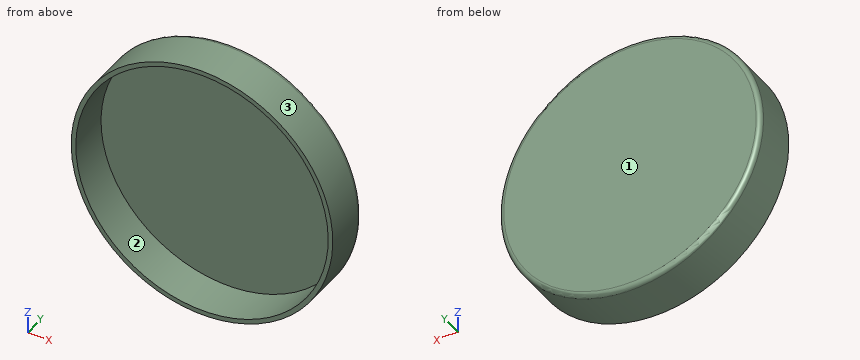
```python
from build123d import *

# Parameters (mm, degrees)
ESQUISSE1_R        = 14.3
BOSS_EXTRU_1_DEPTH = 5
COQUE1_T           = -0.5
CONG_1_R           = 0.5


with BuildPart() as part:
    # Esquisse1 → Boss.-Extru.1 (new body)
    with BuildSketch(Plane(origin=(0, 0, 0), x_dir=(1, 0, 0), z_dir=(0, 1, 0))):
        with Locations(Location((0, 0, 0), (0, 0, 270))):
            Circle(ESQUISSE1_R)
    extrude(amount=BOSS_EXTRU_1_DEPTH)

    # Coque1
    coque1_openings = [part.faces().sort_by_distance(p)[0] for p in [
        (0, 0, 0),
    ]]
    offset(amount=COQUE1_T, openings=coque1_openings, kind=Kind.INTERSECTION)

    # Congé1
    cong_1_edges = [part.edges().sort_by_distance(p)[0] for p in [
        (0, 5, -14.3),
    ]]
    fillet(cong_1_edges, radius=CONG_1_R)


solid = part.part
```
Can you work these out from the model? Positions are in its coordinate system, mm. Face numbers are marked on the shaded views. Give positions to 0.01 mm unless a question says otherwise; leave off trailing zeros. Loops run counter-clockwise (first coordinate to the right, second up) from the corner with the lowest first, then second, coordinate; pieces in that order, holes last. Notation, with made-up numbers: M 78.5,50 L 111.5,50 A24 ccw 111.5,74 Z; hole C 1.25,84 d10. An arc over 180 degrees is marked long. Use CSV: the item, a comma, the result in double quotes. Start each with the question number.
1. Imagine slicing it at C-C, the plane x = 0. Write out the boundary of the cut face in (y, z), plus the area to 3 significant figures.
2. If I drill on L1, parallel to X at y = 1.65, z = 0; L2, parallel to Y at x = -9, z = -5; L3, parallel to X at y = 1.35, z = 9, over which ranges is the centre line in solid material (lowest first)?
3. Imagine slicing it at A-A, the plane z = 0. Write out the boundary of the cut face in (x, y), plus the area to 3 significant figures.
4. If we mould it in two halves opening along X, with no side actions, what happens to the marked faces 1, 2 and 3? For each: released by +X, released by -X, zero draft, split by the parting line, or undercut.
5. For P1, Ø2, axis at x = -9, y = 2.5, coming from the +Z side; P2, Ø1.5, axis at x = 4, y = 3, coming from the -Z side; P3, Ø3, axis at y = 3, z = -3.5, coming from the +X side, each with a flat end and sliding along its axis, tell me the tip position at first contact or that it passes through.
6. Imagine slicing it at B-B, the plane y = 3.05. Write out the boundary of the cut face in (x, z).
Response values:
1,outline,"M 0,-14.3 L 4.5,-14.3 A0.5 ccw 5,-13.8 L 5,13.8 A0.5 ccw 4.5,14.3 L 0,14.3 L 0,13.8 L 4.5,13.8 L 4.5,-13.8 L 0,-13.8 Z"
1,area,"18.7 mm^2"
2,L1,"-14.3 to -13.8, 13.8 to 14.3"
2,L2,"4.5 to 5"
2,L3,"-11.11 to -10.46, 10.46 to 11.11"
3,outline,"M -14.3,0 L -13.8,0 L -13.8,4.5 L 13.8,4.5 L 13.8,0 L 14.3,0 L 14.3,4.5 A0.5 ccw 13.8,5 L -13.8,5 A0.5 ccw -14.3,4.5 Z"
3,area,"18.7 mm^2"
4,face 1,"zero draft"
4,face 2,"undercut"
4,face 3,"split by the parting line"
5,P1,"z = 11.85"
5,P2,"z = -13.93"
5,P3,"x = 14.16"
6,outline,"C 0,0 d28.6; hole C 0,0 d27.6"
